Geometry: final body of the model. Coordinates: model frame, mm. A direction names the side the tool comes from. Give positions to 0.01 mm unless a question says otherwise; leave off trailing zeros. Order: outer loops, then holes, each group sorted by start corner. A loop starts at its lowest first (then second) coordinate and runs counter-clockwise, first axis right, second up. Notation, with made-up numbers: (37, 69) - (64, 69) arc R8 cw to (64, 83) - close; hole circle Ø8 at (26.5, 63.5). An arc over 180 degrees is marked (long way). Put each result on its own line as item: value. Start each with the question number.
1. Mould query, pull axis X, two halves, no side actions, for faces 1 (the flat face through (-30, -35, 5)), 2 (the flat face through (-165.836, -30.551, 27.428)), 3 (the cylindrical face through (-164, -50, 35)). Classes: pulls with the +X half, pulls with the -X half, needs draft (parallel to the pull), parting line crosses it, or undercut.
2. Section D-D on y = -16.5. Return the cut outline in (x, z), plus the area to 3 significant figures.
3. Section A-A on x = -51.5. Return the cut outline in (y, z), plus the area to 3 significant figures.
4. Ray query, line 1 along Z through (x, y) = (-88, -52); line 2 along X through (y, z) = (-53.5, 49.5); line 3 along X through (y, z) = (-59, 58.5) (3 decimals). Return the intervals inside material, ascending. Write a range as from..to.
5. Set-up query: faces 4 (the flat face through (-30, -45, 5)), 5 (the flat face through (-66, -39, 10)), 6 (the flat face through (-142.56, -39.44, 27.39)), 7 (the cylindrical face through (-6.014, -5.703, 5.07)), 8 (the flat face through (-112, 0, 11)). Return all of +Z, -Z, +X, -X, +Y, -Y with unobstructed straight access to the full face (end or side cutting, diameter ignored); none if empty.
6. First-contact query: P1, Ø6, axis at x = -109, y = -34, coming from the +Z side; P2, Ø1, axis at y = -12, z = 67, coming from the -X side; P3, Ø12, axis at y = -29.5, z = 9.5, coming from the -X side. Flat tips, straight axial feed; report the tip coordinate or a pass-through.
7. Section C-C on x = -89.5. Return the cut outline in (y, z), plus the area to 3 significant figures.
8. Section B-B on y = -24.5. Return the cut outline in (x, z), plus the area to 3 significant figures.
from build123d import *

# Parameters (mm, degrees)
F1_DEPTH = 80
F2_R     = 39.99999
F3_R     = 10
F4_DEPTH = 45
F6_DEPTH = 25
F7_R     = 20


# Not quite as in the source:
# - a fillet or chamfer is up to 0.001 mm smaller than in the source, because OpenCascade refuses the exact size


with BuildPart() as f1:
    # F0 (on Front) → F1 (new body)
    with BuildSketch(Plane.XZ):
        Polygon((-150, 0), (0, 0), (0, 10), (-109.5854811567, 10), (-155.3589838486, 89.2820323028), (-164.0192378865, 84.2820323028), (-134.0192378865, 32.3205080757), (-151.3397459622, 22.3205080757), (-181.3397459622, 74.2820323028), (-190, 69.2820323028), align=None)
    extrude(amount=F1_DEPTH)

    # F2 (radius 40 in the source; OpenCascade refuses exactly that, so slightly less here)
    f2_edges = [f1.edges().sort_by_distance(p)[0] for p in [
        (-159.689111, -80, 86.782032),
        (-159.689111, 0, 86.782032),
        (-185.669873, -80, 71.782032),
        (-185.669873, 0, 71.782032),
    ]]
    fillet(f2_edges, radius=F2_R)

    # F3 (on face) → F4 (cut)
    with BuildSketch(Plane(origin=(-77.8589838486, 0, -44.9519052838), x_dir=(0, 1, 0), z_dir=(0.8660254038, 0, 0.5))):
        with Locations((-40, 112.1529946162)):
            Circle(F3_R)
    extrude(amount=-F4_DEPTH, mode=Mode.SUBTRACT)

    # F5 (on face) → F6 (cut)
    with BuildSketch(Plane.XY.offset(10)):
        with BuildLine():
            Line((0, -40), (0, -35))
            Line((0, -35), (-60, -35))
            ThreePointArc((-60, -35), (-56.4644660941, -36.4644660941), (-55, -40))
            Line((-55, -40), (0, -40))
        make_face()
        with BuildLine():
            ThreePointArc((-55, -40), (-56.4644660941, -36.4644660941), (-60, -35))
            ThreePointArc((-60, -35), (-65, -40), (-60, -45))
            ThreePointArc((-60, -45), (-56.4644660941, -43.5355339059), (-55, -40))
        make_face()
        with BuildLine():
            Line((0, -45), (0, -40))
            Line((0, -40), (-55, -40))
            ThreePointArc((-55, -40), (-56.4644660941, -43.5355339059), (-60, -45))
            Line((-60, -45), (0, -45))
        make_face()
    extrude(amount=-F6_DEPTH, mode=Mode.SUBTRACT)

    # F7
    f7_edges = [f1.edges().sort_by_distance(p)[0] for p in [
        (0, -80, 5),
        (0, 0, 5),
    ]]
    fillet(f7_edges, radius=F7_R)


solid = f1.part
Resolved:
1. face 1: needs draft
1. face 2: pulls with the -X half
1. face 3: undercut
2. outline: (-186.18, 62.67) - (-150, 0) - (-0.31, 0) - (-0.31, 10) - (-109.59, 10) - (-151.54, 82.67) - (-160.2, 77.67) - (-134.02, 32.32) - (-151.34, 22.32) - (-177.52, 67.67) - close
2. area: 3,370 mm^2
3. outline: (-80, 0) - (-45, 0) - (-45, 10) - (-80, 10) - close; (-35, 0) - (0, 0) - (0, 10) - (-35, 10) - close
3. area: 700 mm^2
4. line 1: 0..10
4. line 2: -178.58..-167.03, -143.94..-132.39
4. line 3: -183.775..-172.228, -149.134..-137.587
5. face 4: +Z, -Z, +X
5. face 5: +Z, +X, +Y, -Y
5. face 6: +Y, -Y
5. face 7: +Z, -Z, +X, +Y
5. face 8: +Z, -Z, +X, -X, +Y
6. P1: z = 14.18
6. P2: x = -154.33
6. P3: x = -158.95
7. outline: (-80, 0) - (0, 0) - (0, 10) - (-80, 10) - close
7. area: 800 mm^2
8. outline: (-188.44, 66.58) - (-150, 0) - (0, 0) - (0, 10) - (-109.59, 10) - (-153.8, 86.58) - (-162.46, 81.58) - (-134.02, 32.32) - (-151.34, 22.32) - (-179.78, 71.58) - close
8. area: 3,470 mm^2
